Read the model definition and answer for the solid it produces. Units are mm, in the model's axes. Face numbers are marked on the shaded views. Coordinates: 2 decimals unless noted, no trailing zeros. Order: outer loops, then holes, each group sorted by start corner. A loop starts at its lowest first (then second) coordinate and runs counter-clockwise, first axis right, second up. Notation, with made-up numbers: M 88.5,71.5 L 92.5,71.5 A20 ccw 92.5,81.5 Z; hole C -23.75,-19 d5. An arc over 180 degrees is marked long. Put each result on its own line as item: value.
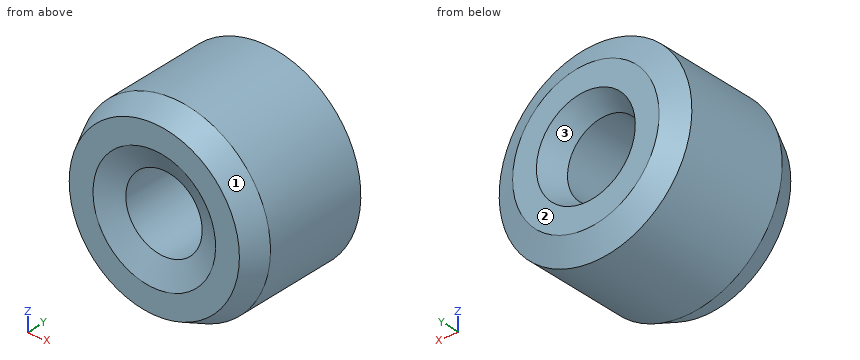
from build123d import *
from OCP.BRepFilletAPI import BRepFilletAPI_MakeChamfer

# Parameters (mm, degrees)
SKETCH1_R           = 12.5
BOSS_EXTRUDE1_DEPTH = 18.094022
SKETCH2_R           = 4.955152252
CUT_EXTRUDE1_DEPTH  = 26.296118914
CHAMFER1_SIZE       = 2.997965
CHAMFER1_SIZE2      = 1.460521


with BuildPart() as part:
    # Sketch1 → Boss-Extrude1 (new body)
    with BuildSketch(Plane(origin=(0, 0, 0), x_dir=(1, 0, 0), z_dir=(0, 1, 0))):
        with Locations(Location((0, 0, 0), (0, 0, 270))):
            Circle(SKETCH1_R)
    extrude(amount=BOSS_EXTRUDE1_DEPTH)

    # Sketch2 → Cut-Extrude1 (cut, through all)
    with BuildSketch(Plane(origin=(0, 0, 0), x_dir=(1, 0, 0), z_dir=(0, 1, 0))):
        with Locations(Location((0, 0, 0), (0, 0, 270))):
            Circle(SKETCH2_R)
    extrude(amount=CUT_EXTRUDE1_DEPTH, mode=Mode.SUBTRACT)

    # Chamfer1: one chamfer whose edges measure the first distance from different faces: ONE call of the kernel's chamfer builder (chamfer() names one face for all edges)
    chamfer1_edges_1 = [part.edges().sort_by_distance(p)[0] for p in [
        (0, 0, -12.5),
    ]]
    chamfer1_side_1 = [part.faces().sort_by_distance(p)[0] for p in [
        (0, 9.047011, -12.5),
    ]]
    chamfer1_edges_2 = [part.edges().sort_by_distance(p)[0] for p in [
        (0, 18.094022, -12.5),
    ]]
    chamfer1_side_2 = [part.faces().sort_by_distance(p)[0] for p in [
        (0, 18.094022, -12.146446609),
    ]]
    chamfer1_edges_3 = [part.edges().sort_by_distance(p)[0] for p in [
        (0, 0, -4.955152252),
    ]]
    chamfer1_side_3 = [part.faces().sort_by_distance(p)[0] for p in [
        (0, 0, -12.146446609),
    ]]
    chamfer1_edges_4 = [part.edges().sort_by_distance(p)[0] for p in [
        (0, 18.094022, -4.955152252),
    ]]
    chamfer1_side_4 = [part.faces().sort_by_distance(p)[0] for p in [
        (0, 9.047011, -4.955152252),
    ]]
    chamfer1 = BRepFilletAPI_MakeChamfer(part.part.solid().wrapped)
    for e in chamfer1_edges_1:
        chamfer1.Add(CHAMFER1_SIZE, CHAMFER1_SIZE2, e.wrapped, chamfer1_side_1[0].wrapped)  # the first distance lies on this face
    for e in chamfer1_edges_2:
        chamfer1.Add(CHAMFER1_SIZE, CHAMFER1_SIZE2, e.wrapped, chamfer1_side_2[0].wrapped)  # the first distance lies on this face
    for e in chamfer1_edges_3:
        chamfer1.Add(CHAMFER1_SIZE, CHAMFER1_SIZE2, e.wrapped, chamfer1_side_3[0].wrapped)  # the first distance lies on this face
    for e in chamfer1_edges_4:
        chamfer1.Add(CHAMFER1_SIZE, CHAMFER1_SIZE2, e.wrapped, chamfer1_side_4[0].wrapped)  # the first distance lies on this face
    add(Compound.cast(chamfer1.Shape()), mode=Mode.REPLACE)


solid = part.part
Q1. Find section C-C on y = 11.25. Write down the section's boundary in (x, z), plus the area to 3 significant figures.
Answers below:
outline: C 0,0 d25; hole C 0,0 d9.91
area: 414 mm^2
Q2. For a pull along X with two mould halves and no side action, classify the marked faces 1, 2 and 3 as +X half, -X half, draft (parallel to the pull), parting line (faces both ways), or undercut.
Answers below:
face 1: parting line
face 2: draft
face 3: undercut
Q3. Given pin 1 (8 mm diameter, centred on y = 12, z = 7.5, fed in from -X); pin 2 (11.5 mm diameter, centred on x = 0, z = 0, fed in from +Y); pin 3 (8 mm diameter, centred on x = -8, y = 15.5, fed in from +Z), each flat-ended and moving along its own axis, determine where each tip first touches the part or whether it passes through.
Answers below:
pin 1: stops at x = -12
pin 2: stops at y = 16.73
pin 3: stops at z = 11.84
Q4. Find section B-B on z = 0. Write down the section's boundary in (x, y), plus the area to 3 significant figures.
Answers below:
outline: M -12.5,3 L -11.04,0 L -7.95,0 L -4.96,1.46 L -4.96,15.1 L -6.42,18.09 L -9.5,18.09 L -12.5,16.63 Z; M 4.96,1.46 L 7.95,0 L 11.04,0 L 12.5,3 L 12.5,16.63 L 9.5,18.09 L 6.42,18.09 L 4.96,15.1 Z
area: 256 mm^2
Q5. Find section A-A on x = 0. Write down the section's boundary in (y, z).
Answers below:
outline: M 0,-11.04 L 3,-12.5 L 16.63,-12.5 L 18.09,-9.5 L 18.09,-6.42 L 15.1,-4.96 L 1.46,-4.96 L 0,-7.95 Z; M 0,7.95 L 1.46,4.96 L 15.1,4.96 L 18.09,6.42 L 18.09,9.5 L 16.63,12.5 L 3,12.5 L 0,11.04 Z
Q6. Consider line 1 along X through (y, z) = (9.5, 0); line 2 along Z through (x, y) = (1.25, 12.75); line 3 along Z through (x, y) = (-5, 16.5). Determine where each line is inside the solid, lowest interval first.
Answers below:
line 1: x = -12.5 to -4.96, 4.96 to 12.5
line 2: z = -12.44 to -4.79, 4.79 to 12.44
line 3: z = -11.46 to -2.61, 2.61 to 11.46
